Verification items for the finished model (mm, model axes). A direction names the side the tool comes from. Coordinates: 2 decimals unless noted, no trailing zeros. Write each loop counter-clockwise with the first axis right and the second up, starting at its lowest first coordinate (ties: lowest second). Pieces come first, ordered by that corner, then holes. Notation, with made-up numbers: (2.5, 66) -> (55.5, 66) arc R18 ccw to (55.5, 89) -> close; hole circle Ø4 at (17.25, 69). An arc over 180 degrees is marked (long way). Use CSV: the item, a comma, the result in double quotes.
Autodesk Inventor part; units mm, degrees
ref_plane "YZ Plane" through (0, 0, 0) normal (1, 0, 0) x (0, 1, 0)
ref_plane "XZ Plane" through (0, 0, 0) normal (0, 1, 0) x (-1, 0, 0)
ref_plane "XY Plane" through (0, 0, 0) normal (0, 0, 1) x (1, 0, 0)
sketch "Sketch1" plane through (0, 0, 0) normal (0, 1, 0) x (-1, 0, 0)
  line L0 (12.35, 8.5) -> (-12.35, 8.5)
  line L1 (-12.35, 8.5) -> (-12.35, -8.5)
  line L2 (-12.35, -8.5) -> (12.35, -8.5)
  line L3 (12.35, -8.5) -> (12.35, 8.5)
  line L4 (12.35, 8.5) -> (-12.35, -8.5) construction
  line L5 (-12.35, 8.5) -> (12.35, -8.5) construction
  point P0 (0, 0)
  dimension "d0" = 24.7
  dimension "d1" = 17
extrude "Extrusion1" add sketch "Sketch1" along normal blind 10
sketch "Sketch2" plane through (0, 10, 0) normal (0, 1, 0) x (1, 0, 0)
  line L0 (-12.35, 8.1) -> (12.35, 8.1)
  line L1 (12.35, 8.1) -> (12.35, -8.1)
  line L2 (12.35, -8.1) -> (-12.35, -8.1)
  line L3 (-12.35, -8.1) -> (-12.35, 8.1)
  line L4 (-12.35, 8.1) -> (12.35, -8.1) construction
  line L5 (12.35, 8.1) -> (-12.35, -8.1) construction
  point P0 (0, 0)
  dimension "d4" = 24.7
  dimension "d5" = 16.2
extrude "Extrusion2" cut sketch "Sketch2" against normal blind 9
sketch "Sketch3" plane through (0, 0, 0) normal (0, -1, 0) x (1, 0, 0)
  line L0 (-12.35, -8.5) -> (-12.35, 8.5)
  line L1 (12.35, 8.5) -> (12.35, -8.5)
  line L2 (-12.35, 0) -> (-9.35, 0)
  circle A0 centre (-9.35, 0) radius 1.5
  line L3 (12.35, 0) -> (9.35, 0)
  circle A1 centre (9.35, 0) radius 1.5
  point P0 (0, 0)
  dimension "d8" = 3
  dimension "d9" = 3
  dimension "d10" = 3
  dimension "d11" = 3
extrude "Extrusion3" cut sketch "Sketch3" against normal blind 1
sketch "Sketch4" plane through (-12.35, 0, -8.5) normal (-1, 0, 0) x (0, 0, 1)
  line L0 (0.4, 1) -> (0.4, 10)
  line L1 (0, 10) -> (0.4, 10)
  line L2 (0, 0) -> (0, 10)
  line L3 (0, 0) -> (17, 0)
  line L4 (17, 0) -> (17, 10)
  line L5 (16.6, 10) -> (17, 10)
  line L6 (16.6, 10) -> (16.6, 1)
  line L7 (16.6, 1) -> (0.4, 1)
  point P0 (8.5, 0)
extrude "Extrusion4" add sketch "Sketch4" along normal blind 2
sketch "Sketch5" plane through (-14.35, 0, -8.5) normal (-1, 0, 0) x (0, 0, 1)
  line L0 (0.4, 1) -> (0.4, 10)
  line L1 (0.4, 10) -> (0, 10)
  line L2 (0, 10) -> (0, 0)
  line L3 (0, 0) -> (17, 0)
  line L4 (17, 0) -> (17, 10)
  line L5 (17, 10) -> (16.6, 10)
  line L6 (16.6, 10) -> (16.6, 1)
  line L7 (16.6, 1) -> (0.4, 1)
  point P0 (8.5, 0)
extrude "Extrusion5" cut sketch "Sketch5" against normal blind 0.2
sketch "Sketch6" plane through (0, 0, 0) normal (0, -1, 0) x (1, 0, 0)
  line L0 (-14.15, 8.5) -> (-14.15, -8.5)
  line L1 (-14.15, 8.5) -> (12.35, 8.5)
  circle A0 centre (-9.35, 0) radius 1.5
  line L2 (-14.15, 0) -> (-12.15, 0)
  line L3 (-12.15, 0) -> (-10.15, 0)
  line L4 (-10.15, 0) -> (-7.15, 0)
  point P0 (0, 0)
  dimension "d18" = 2
  dimension "d19" = 2
  dimension "d20" = 3
extrude "Extrusion6" add sketch "Sketch6" against normal blind 1
sketch "Sketch7" plane through (0, 0, 0) normal (0, -1, 0) x (1, 0, 0)
  line L0 (-14.15, 8.5) -> (-14.15, -8.5)
  line L1 (-14.15, 8.5) -> (12.35, 8.5)
  line L2 (-14.15, 0) -> (-10.85, 0)
  line L3 (-10.85, 0) -> (-7.85, 0)
  circle A0 centre (-7.85, 0) radius 1.5
  point P0 (0, 0)
  dimension "d29" = 3.3
  dimension "d30" = 3
  dimension "d31" = 3
extrude "Extrusion7" cut sketch "Sketch7" against normal blind 1
sketch "Sketch8" plane through (0, 1, 0) normal (0, 1, 0) x (1, 0, 0)
  circle A0 centre (-7.85, 0) radius 1.5
  circle A1 centre (9.35, 0) radius 1.5
  circle A2 centre (9.35, 0) radius 0.05
  circle A3 centre (-7.85, 0) radius 0.05
  point P0 (0, 0)
  dimension "d34" = 0.1
  dimension "d35" = 0.1
extrude "Extrusion8" add sketch "Sketch8" against normal blind 1
sketch "Sketch9" plane through (0, 1, 0) normal (0, 1, 0) x (1, 0, 0)
  circle A0 centre (-7.85, 0) radius 0.05
  circle A1 centre (9.35, 0) radius 0.05
  circle A2 centre (-7.85, 0) radius 1.5
  circle A3 centre (9.35, 0) radius 1.5
  point P0 (0, 0)
  dimension "d38" = 3
  dimension "d39" = 3
extrude "Extrusion9" cut sketch "Sketch9" against normal blind 1
properties part number "kolejnicka_ruka"
1) Cross-section at C-C (y = 6.5). Record the boundary of the cut face in (x, z), plus the area to 3 significant figures.
Return value:
outline,"(-14.15, -8.5) -> (12.35, -8.5) -> (12.35, -8.1) -> (-14.15, -8.1) -> close; (-14.15, 8.1) -> (12.35, 8.1) -> (12.35, 8.5) -> (-14.15, 8.5) -> close"
area,"21.2 mm2"
2) Set-up check for faces 1 (the flat face through (-14.15, 0.6, 0)), 2 (the flat face through (-1, 1, 0)): record each of +Z, -Z, +X, -X, +Y, -Y from which the full face is reachable in a straight line by a thin tool's end or side.
Return value:
face 1,"+Z, -Z, -X, +Y, -Y"
face 2,"+X, -X, +Y"
3) Mould release check, pull along X, two halves, no side actions. Record for faces 3 (the flat face through (12.35, 0.5, 0)), 4 (the flat face through (-1, 5, -8.1)), 5 (the cylindrical face through (10.736, 0.507, 0.575)): released by +X, released by -X, zero draft, split by the parting line, or undercut.
Return value:
face 3,"released by +X"
face 4,"zero draft"
face 5,"undercut"
4) Cross-section at D-D (x = -2.25). Record the boundary of the cut face in (y, z), plus the area to 3 significant figures.
Return value:
outline,"(0, -8.5) -> (10, -8.5) -> (10, -8.1) -> (1, -8.1) -> (1, 8.1) -> (10, 8.1) -> (10, 8.5) -> (0, 8.5) -> close"
area,"24.2 mm2"
5) Gauge pin test, flat end, axial feed: pin 1 (3.5 mm diameter, centred on x = -7.85, z = 0, fed in from +Y). Record the tip position at first contact, or that the pin passes through.
Return value:
pin 1,"y = 1"
6) Cross-section at B-B (z = 0). Record the boundary of the cut face in (x, y), plus the area to 3 significant figures.
Return value:
outline,"(-14.15, 0) -> (-9.35, 0) -> (-9.35, 1) -> (-14.15, 1) -> close; (-6.35, 0) -> (7.85, 0) -> (7.85, 1) -> (-6.35, 1) -> close; (10.85, 0) -> (12.35, 0) -> (12.35, 1) -> (10.85, 1) -> close"
area,"20.5 mm2"
7) Scan lines: L1, parallel to X at y = 0.55, z = 0; L2, parallel to Z at x = -7.85, y = 0.4; L3, parallel to Z at x = 8.5, y = 8.25. Record each from-to range of solid material in increasing order.
Return value:
L1,"-14.15 to -9.35, -6.35 to 7.85, 10.85 to 12.35"
L2,"-8.5 to -1.5, 1.5 to 8.5"
L3,"-8.5 to -8.1, 8.1 to 8.5"
8) Cross-section at A-A (x = -7.85). Record the boundary of the cut face in (y, z).
Return value:
outline,"(0, -8.5) -> (10, -8.5) -> (10, -8.1) -> (1, -8.1) -> (1, -1.5) -> (0, -1.5) -> close; (0, 1.5) -> (1, 1.5) -> (1, 8.1) -> (10, 8.1) -> (10, 8.5) -> (0, 8.5) -> close"
